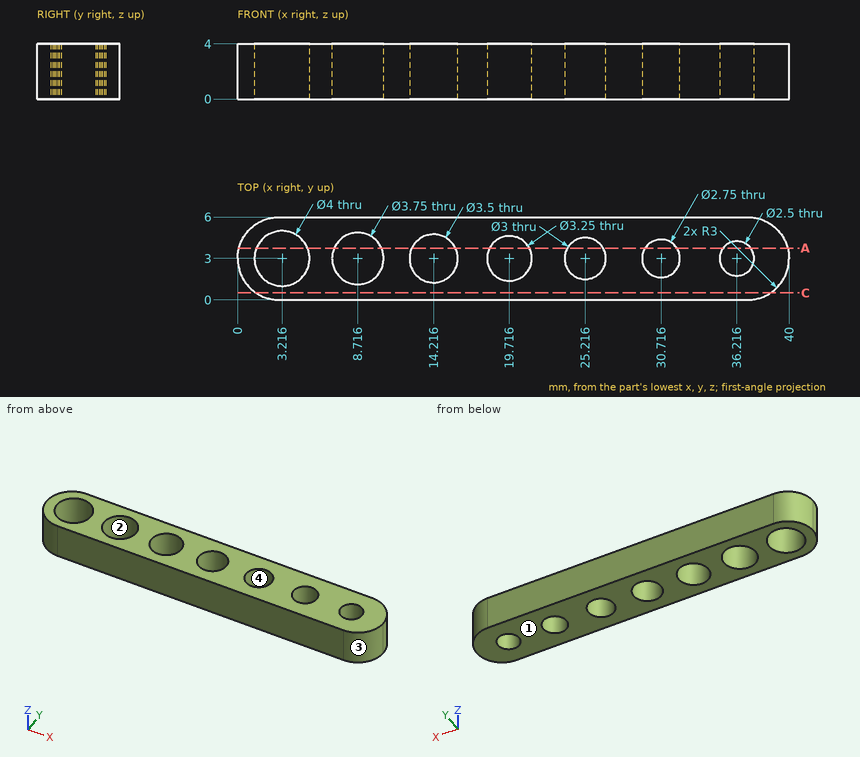
Could you check a few things on this drawing? It's one solid part, dimensions in mm from its lowest x, y, z. Round coordinates to 2 decimals unless told otherwise and drop trailing zeros. Write each loop counter-clockwise with the first axis right and the second up, starting at its lowest first coordinate (ties: lowest second). Pieces come first, ordered by that corner, then holes.
Q1. If we section it at C-C on y = 0.5: Write out the boundary of the cut face in (x, z).
Q2. Will this pin go through, and if not, where does the flat tip stop? P1, Ø1.5, axis at y = 5, z = 2, coming from the -X side.
Q3. If we section it at A-A on y = 3.75: Give the number of separate pieces and of enclosed holes in the cut face.
Q4. Please list where these lines run through material, in increasing order: probe 1 along Y at (x, z) = (14, 1.7); probe 2 along Y at (x, z) = (3.5, 2.05); probe 3 along X at (y, z) = (5.5, 2).
Q5. If we mould it in two halves opening along Y, with no side actions, what happens to the marked faces 1, 2, 3 and 4? For each: +Y half, -Y half, draft (parallel to the pull), parting line (faces both ways), or undercut.
Answer below:
1. outline: (1.34, 0) - (38.66, 0) - (38.66, 4) - (1.34, 4) - close
2. P1: stops at x = 0.27
3. separate pieces: 8
3. enclosed holes: 0
4. probe 1: y = 0 to 1.26, 4.74 to 6
4. probe 2: y = 0 to 1.02, 4.98 to 6
4. probe 3: x = 1.34 to 38.66
5. face 1: draft
5. face 2: undercut
5. face 3: -Y half
5. face 4: undercut
